Autodesk Inventor part; units mm, degrees
ref_plane "YZ Plane" through (0, 0, 0) normal (1, 0, 0) x (0, 1, 0)
ref_plane "XZ Plane" through (0, 0, 0) normal (0, 1, 0) x (-1, 0, 0)
ref_plane "XY Plane" through (0, 0, 0) normal (0, 0, 1) x (1, 0, 0)
sketch "Sketch1" plane through (0, 0, 0) normal (0, 0, 1) x (1, 0, 0)
  line L0 (0, 25.4) -> (-28.702, 25.4) construction
  line L1 (0, 25.4) -> (-95.25, 25.4) construction
  line L2 (-95.25, 25.4) -> (-90.805, 25.4) construction
  line L3 (-90.805, 25.4) -> (-90.805, 22.4389) construction
  line L4 (-90.805, 0) -> (-95.25, 0)
  line L5 (-28.702, 59.6457) -> (-28.702, -91.9304) construction
  arc A0 (-28.9184, -9.248) -> (-32.3684, -1.8494) centre (-35.052, -7.6045) ccw
  line L6 (-76.2, -185.7054) -> (-28.702, -8.4405)
  line L7 (-90.805, 25.4) -> (-90.805, 0)
  line L8 (-87.63, 23.9195) -> (-32.3684, -1.8494)
  line L9 (-28.702, -7.6045) -> (-60.452, -7.6045) construction
  line L10 (-60.452, -126.9331) -> (-54.102, -126.9331) construction
  line L11 (-54.102, -126.9331) -> (-54.102, -103.2346) construction
  line L12 (-54.102, -103.2346) -> (-60.452, -103.2346)
  line L13 (-60.452, 11.2462) -> (-60.452, 1.7212) construction
  line L14 (-60.452, 11.2462) -> (-60.452, 4.7154) construction
  line L15 (-60.452, 4.7154) -> (-46.4468, 4.7154)
  line L16 (-95.25, 0) -> (-95.25, -12.7) construction
  line L17 (-60.452, -12.7) -> (-73.152, -12.7) construction
  line L18 (-95.25, -12.7) -> (-95.25, -25.4) construction
  line L19 (-95.25, -25.4) -> (-95.25, -88.9) construction
  line L20 (-95.25, -88.9) -> (-82.55, -88.9) construction
  line L21 (-82.55, -88.9) -> (-82.55, -25.4) construction
  line L22 (-95.25, -25.4) -> (-82.55, -25.4)
  line L23 (-82.55, -25.4) -> (-82.55, -88.9)
  line L24 (-82.55, -88.9) -> (-95.25, -88.9)
  line L25 (-95.25, -12.7) -> (-73.152, -12.7)
  line L26 (-73.152, -138.7824) -> (-63.627, -138.7824)
  line L27 (-82.55, -88.9) -> (-82.55, -185.7054)
  line L28 (-82.55, -185.7054) -> (-76.2, -185.7054)
  line L29 (-73.152, -12.7) -> (-73.152, -138.7824)
  line L30 (-88.9, -25.4) -> (-88.9, -31.3436)
  line L31 (-88.9, -31.3436) -> (-95.25, -31.3436)
  line L32 (-95.25, 0) -> (-95.25, -25.4)
  line L33 (-95.25, -31.3436) -> (-95.25, -88.9)
  line L34 (-88.9, -160.3054) -> (-88.9, -221.2532)
  line L35 (-28.9184, -9.248) -> (-85.725, -221.2532)
  line L36 (-85.725, -221.2532) -> (-88.9, -221.2532)
  line L37 (-82.55, -160.3054) -> (-88.9, -160.3054)
  line L38 (-66.802, -38.1) -> (-66.802, 4.7154)
  line L39 (-66.802, 4.7154) -> (-60.452, 4.7154)
  line L40 (-66.802, -38.1) -> (-60.452, -103.2346)
  line L41 (-60.452, 11.2462) -> (-60.452, 4.7154) construction
  line L42 (-60.452, -7.6045) -> (-60.452, -12.7) construction
  line L43 (-60.452, -103.2346) -> (-60.452, -126.9331) construction
  line L44 (0, 59.6457) -> (0, -91.9304) construction
  line L45 (-73.152, -38.1) -> (-69.977, -38.1)
  line L46 (-69.977, -38.1) -> (-69.977, -12.7)
  line L47 (-66.802, -12.7) -> (-69.977, -12.7)
  line L48 (-90.805, 25.4) -> (-87.63, 25.4)
  line L49 (-87.63, 25.4) -> (-87.63, 23.9195)
  point P0 (0, 0)
  point P1 (-95.25, -255.9127)
  point P2 (-88.7095, 22.4389)
  dimension "d0" = 28.702
  dimension "d1" = 95.25
  dimension "d2" = 4.445
  dimension "d5" = 25.4
  dimension "d6" = 25.4
  dimension "d8" = 12.7
  dimension "d12" = 31.75
  dimension "d13" = 6.35
  dimension "d16" = 12.7
  dimension "d17" = 12.7
  dimension "d18" = 12.7
  dimension "d19" = 63.5
  dimension "d20" = 12.7
  dimension "d22" = 9.525
  dimension "d23" = 6.35
  dimension "d25" = 5.9436
  dimension "d27" = 3.175
  dimension "d28" = 6.35
  dimension "d29" = 25.4
  dimension "d30" = 107.95
  dimension "d31" = 6.35
  dimension "d33" = 20.3552
  dimension "d34" = 15
  dimension "d35" = 3.175
  dimension "d36" = 25.4
  dimension "d38" = 3.175
  dimension "d39" = 1.4805
  dimension "d40" = 25
revolve "Revolution1" add sketch "Sketch1" angle 360 about axis through (0, 59.6457, 0) along (0, -1, 0) contours L7 L48 L49 L8 L15 L39 L38 L47 L46 L45 L29 L25 L32 L4
properties part number "phenolic_top" material "Phenolic Resin"
Could you check a few things on this model? Use its own coordinates, in mm. A direction names the side the tool comes from. Round coordinates to 2 decimals unless told otherwise and drop trailing zeros. Order: outer loops, then holes, each group sorted by start corner. A loop starts at its lowest first (then second) coordinate and runs counter-clockwise, first axis right, second up.
Q1. Please list where these lines run through material, in increasing order: probe 1 along X at (y, z) = (-22, 0); probe 2 along Z at (x, y) = (0, 24.75) (3 decimals).
Geometry says:
probe 1: x = -73.15 to -69.98, 69.98 to 73.15
probe 2: z = -90.805 to -87.63, 87.63 to 90.805
Q2. Thinking about a two-plate mould opening in Z: for faces 4 (the face through (75.587, -6.439, 57.958)), 5 (the face through (-84, 0, 35)), 6 (the face through (10.63, 5.92, -47.86)), which applies, released by +Z, released by -Z, zero draft, split by the parting line, or undercut?
Geometry says:
face 4: split by the parting line
face 5: zero draft
face 6: undercut
Q3. Imagine slicing it at B-B, the plane y = -22.5. List the corners of the cut face in (x, z) for me.
Geometry says:
outline: circle Ø146.3 at (0, 0); hole circle Ø139.95 at (0, 0)
Q4. Which directions (+Z, -Z, +X, -X, +Y, -Y) give clear straight access to the entire face, cutting with the end or side of a thin tool? Please do faces 1 (the face through (14.481, -3.87, -65.213)), 2 (the face through (48, 25.4, -74)), 3 (the face through (-86.61, 12.52, -27.28)).
Geometry says:
face 1: -Y
face 2: +Z, -Z, +X, -X, +Y
face 3: +Y
Q5. Imagine slicing it at D-D, the plane y = 18. List the corners of the cut face in (x, z) for me (3 decimals), then the cut area to 3 significant figures.
Geometry says:
outline: circle Ø181.61 at (0, 0); hole circle Ø149.871 at (0, 0)
area: 8,260 mm2
Q6. I'm going to push flat-ended pins straight in: P1, Ø3, axis at x = -12.5, z = -51.5, coming from the +Y side; P2, Ø2, axis at x = 46, z = 13, coming from the -Y side; P3, Ø6, axis at y = 7, z = 52, coming from the -X side. Where does each tip first touch, or does it pass through?
Geometry says:
P1: stops at y = 8.47
P2: stops at y = 4.72
P3: stops at x = -76.45
